The model under review builds one solid part; all positions refer to its coordinate system, in mm. A direction names the side the tool comes from. Round coordinates to 2 decimals unless told otherwise and drop trailing zeros. Order: outer loops, then holes, each group sorted by start corner. A loop starts at its lowest first (then second) coordinate and runs counter-clockwise, first axis right, second up. Notation, with made-up numbers: M -26.5,31.5 L -17.5,31.5 A29 ccw -17.5,69.5 Z; hole C -30.5,33.5 d11. An arc over 180 degrees is marked long. Use a Markdown table: item, result. Add a question column.
1. To check wall thickness, follow probe 1 along X at (y, z) = (5.75, -9); probe 2 along Z at (x, y) = (6.5, 0.5); probe 3 along Z at (x, y) = (-1, 4). State the ranges of each line that lie inside material, in increasing order.
2. Consider section A-A on x = -19. State the section outline as (y, z) points.
3. The part is to be moulded in two halves that separate along Z. For faces 1 (the flat face through (-21, 0, 66)), 2 (the cylindrical face through (-61.82, 3.13, -80.63)), 3 (the cylindrical face through (20.027, 3.131, 63.596)), say which applies: +Z half, -Z half, draft (parallel to the pull), parting line (faces both ways), or undercut.
4. For faces 4 (the cylindrical face through (-71.82, 4.48, -43.14)), 5 (the cylindrical face through (46.647, 1.257, 67.943)), list the 3-axis set-ups (+Z, -Z, +X, -X, +Y, -Y) from which the entire face can be reached by the end or side of a thin tool; tool diameter is ignored.
5. Insertion check: P1, Ø9, axis at x = 45.82, z = 70.57, coming from the +Y side; P2, Ø1, axis at y = 0.5, z = -76, coming from the -X side. Each pin has a flat end and moves straight along its axis. Give the tip position at first contact, or say it passes through.
6. Consider section B-B on y = 1.5. Count the separate pieces of the cut face and the enclosed holes in it, then the cut area to 3 significant figures.
from build123d import *

# Parameters (mm, degrees)
SKETCH1_R                                        = 101.6
SKETCH1_R_2                                      = 66.675
SKETCH1_R_3                                      = 0.254
BOSS_EXTRUDE1_DEPTH                              = 6.35
CBORE_FOR_M5_HEX_HEAD_MACHINE_SCREW1_D           = 5.5
CBORE_FOR_M5_HEX_HEAD_MACHINE_SCREW1_CBORE_D     = 11.71
CBORE_FOR_M5_HEX_HEAD_MACHINE_SCREW1_CBORE_DEPTH = 3.8
CIRPATTERN1_COUNT                                = 12


with BuildPart() as part:
    # Sketch1 → Boss-Extrude1 (new body)
    with BuildSketch(Plane(origin=(0, 0, 0), x_dir=(1, 0, 0), z_dir=(0, 1, 0))):
        with Locations(Location((0, 0, 0), (0, 0, 270))):
            Circle(SKETCH1_R)
        with Locations(Location((0, 0, 0), (0, 0, 270))):
            Circle(SKETCH1_R_2, mode=Mode.SUBTRACT)
        with Locations(Location((-74.964980341, 38.201709762, 0), (0, 0, 270))):
            Circle(SKETCH1_R_3, mode=Mode.SUBTRACT)
    extrude(amount=BOSS_EXTRUDE1_DEPTH)

    # CBORE for M5 Hex Head Machine Screw1 (through all)
    with Locations(Plane(origin=(0, 6.35, 0), x_dir=(1, 0, 0), z_dir=(0, 1, 0))):
        with Locations((-74.964980341, 38.201709762)):
            cbore_for_m5_hex_head_machine_screw1 = CounterBoreHole(CBORE_FOR_M5_HEX_HEAD_MACHINE_SCREW1_D / 2, CBORE_FOR_M5_HEX_HEAD_MACHINE_SCREW1_CBORE_D / 2, CBORE_FOR_M5_HEX_HEAD_MACHINE_SCREW1_CBORE_DEPTH)

    # CirPattern1: CBORE for M5 Hex Head Machine Screw1 ×12 about axis
    cirpattern1_axis = Axis((0, 0, 0), (0, 1, 0))
    for i in range(1, CIRPATTERN1_COUNT):
        add(cbore_for_m5_hex_head_machine_screw1.rotate(cirpattern1_axis, i * 360 / CIRPATTERN1_COUNT), mode=Mode.SUBTRACT)


solid = part.part
Answer block:
| question | item | result |
|---|---|---|
| 1 | probe 1 | -101.2 to -66.06, 66.06 to 80.4, 87.64 to 101.2 |
| 1 | probe 2 | -101.39 to -66.36, 66.36 to 82.25, 85.8 to 101.39 |
| 1 | probe 3 | -101.6 to -88.79, -79.25 to -66.67, 66.67 to 81.76, 86.29 to 101.6 |
| 2 | outline | M 0,-99.81 L 6.35,-99.81 L 6.35,-63.91 L 0,-63.91 Z; M 0,63.91 L 6.35,63.91 L 6.35,99.81 L 0,99.81 Z |
| 3 | face 1 | draft |
| 3 | face 2 | parting line |
| 3 | face 3 | undercut |
| 4 | face 4 | +Y |
| 4 | face 5 | +Y, -Y |
| 5 | P1 | y = 2.55 |
| 5 | P2 | x = -67.99 |
| 6 | separate pieces | 1 |
| 6 | enclosed holes | 13 |
| 6 | area | 18,200 mm^2 |
